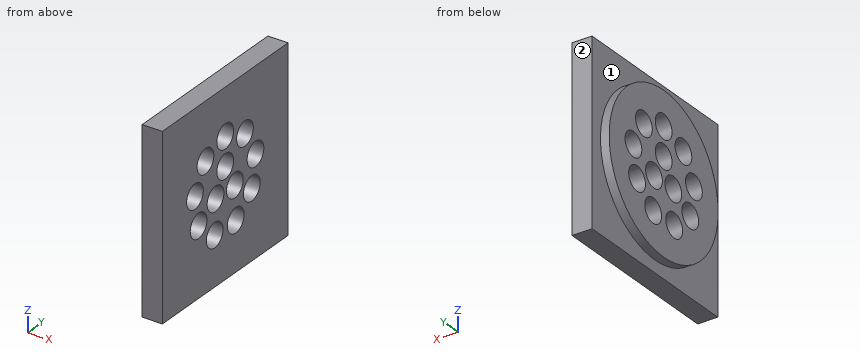
from build123d import *

# Parameters (mm, degrees)
F2_W     = 90
F2_H     = 90
F3_DEPTH = 10
F4_D     = 12
F4_DEPTH = 20
F4_TIP   = 3.6051637142


# Not quite as in the source:
# - a feature names something its author has since deleted; it is built from what else it names


with BuildPart() as f1:
    # F0 (on Front) → F1 (revolve)
    with BuildSketch(Plane.XZ):
        Polygon((-14.3225658685, 0), (-10, 0), (-10, 32.5), (-10, 39), (-14.3225658685, 39), (-14.3225658685, 34.4556160271), (-14.3225658685, 32.5), align=None)
    revolve(axis=Axis((-45.5725640059, 0, 0), (-1, 0, 0)))

    # F2 (on Right) → F3 (join)
    with BuildSketch(Plane.YZ):
        Rectangle(F2_W, F2_H)
    extrude(amount=-F3_DEPTH)

    # F4
    with Locations(Plane.YZ):
        with Locations((-6.9282032303, -4), (6.9282032303, -4), (0, 8), (-21.6657705663, 3.8202599087), (-14.1413274131, 16.8529777486), (0, 22), (14.1413274131, 16.8529777486), (21.6657705663, 3.8202599087), (19.0525588833, -11), (7.5244431532, -20.6732376573), (-7.5244431532, -20.6732376573), (-19.0525588833, -11)):
            Hole(F4_D / 2, depth=F4_DEPTH)
            with Locations((0, 0, -(F4_DEPTH + F4_TIP / 2))):  # 118° drill point
                Cone(0, F4_D / 2, F4_TIP, mode=Mode.SUBTRACT)


solid = f1.part
Geometry: final body of the model. Coordinates: model frame, mm. Face numbers are marked on the shaded views. A direction names the side the tool comes from. Give positions to 0.01 mm unless a question says otherwise; leave off trailing zeros. Loops run counter-clockwise (first coordinate to the right, second up) from the corner with the lowest first, then second, coordinate; pieces in that order, holes last. Notation, with made-up numbers: (-35, 54) -> (12, 54) arc R17 ccw to (12, 61) -> close; hole circle Ø5 at (-35.75, 25). An arc over 180 degrees is marked (long way). Put each result on its own line as item: value.
1. Cut plane B-B (z = -23). Return the cut outline in (x, y).
Taken from the geometry:
outline: (-14.32, -31.5) -> (-10, -31.5) -> (-10, -45) -> (0, -45) -> (0, -13.05) -> (-14.32, -13.05) -> close; (-14.32, -1.99) -> (0, -1.99) -> (0, 1.99) -> (-14.32, 1.99) -> close; (-14.32, 13.05) -> (0, 13.05) -> (0, 45) -> (-10, 45) -> (-10, 31.5) -> (-14.32, 31.5) -> close
2. Set-up query: the marked faces 1 and 2. Return all of +Z, -Z, +X, -X, +Y, -Y with unobstructed straight access to the full face (end or side cutting, diameter ignored); none if empty.
Taken from the geometry:
face 1: -X
face 2: +Z, -Z, +X, -X, +Y
3. Ray query, line 1 along Z through (x, y) = (-9.5, 7); line 2 along Y through (x, z) = (-9.5, -12.5); line 3 along Y through (x, z) = (-4.5, 12). Return the intervals inside material, ascending. Write a range as [from, to].
Taken from the geometry:
line 1: z = [-45, -26.65], [-14.7, -10], [2, 45]
line 2: y = [-45, -24.86], [-13.24, 13.24], [24.86, 45]
line 3: y = [-45, -17.67], [-10.61, -4.47], [4.47, 10.61], [17.67, 45]
4. Pin query (flat end, axial travel): P1, Ø7, axis at y = 14.14, z = 16.85, coming from the +X side. Return the tip coordinate at first contact, or that it passes through.
Taken from the geometry:
P1: passes through
5. Cut plane A-A (z = 8). Return the cut outline in (x, y), plus the area to 3 significant figures.
Taken from the geometry:
outline: (-14.32, -38.17) -> (-10, -38.17) -> (-10, -45) -> (0, -45) -> (0, -25.97) -> (-14.32, -25.97) -> close; (-14.32, -17.36) -> (0, -17.36) -> (0, -6) -> (-14.32, -6) -> close; (-14.32, 6) -> (0, 6) -> (0, 17.36) -> (-14.32, 17.36) -> close; (-14.32, 25.97) -> (0, 25.97) -> (0, 45) -> (-10, 45) -> (-10, 38.17) -> (-14.32, 38.17) -> close
area: 812 mm2
6. Cut plane D-D (y = -30). Return the cut outline in (x, z), plus the area to 3 significant figures.
Taken from the geometry:
outline: (-14.32, -24.92) -> (-10, -24.92) -> (-10, -45) -> (0, -45) -> (0, 45) -> (-10, 45) -> (-10, 24.92) -> (-14.32, 24.92) -> close
area: 1,120 mm2
7. Cut plane C-C (x = -6.5). Count the separate pieces of the cut face and the enclosed holes in it, plus the area to 3 significant figures.
Taken from the geometry:
separate pieces: 1
enclosed holes: 12
area: 6,740 mm2
